Input: part model. Units: mm. Frame: model coordinates. A direction names the side the tool comes from. Coordinates: 2 decimals unless noted, no trailing zeros. Write each loop counter-clockwise with the first axis right and the second up, starting at its lowest first coordinate (ties: lowest second). Pieces come first, ordered by that corner, then holes. Notation, with made-up numbers: (-12.5, 3) - (10.5, 3) arc R37 ccw to (10.5, 41) - close; hole circle Ø1 at (16.25, 47.25). An arc over 180 degrees is marked (long way). Put each result on its own line as item: value. Start each with the question number.
1. Line query: line 1 (X direction, y = -1, z = -26.05); line 2 (Y direction, x = -23.25, z = -18); line 3 (Z direction, x = 24.5, y = -2.5). Output: solid intervals per line, ascending.
2. Cut plane B-B, the plane x = 24.1. Return loops of the section in (y, z), and give its area (3 significant figures).
3. Pin query (flat end, axial travel): pin 1 (4.5 mm diameter, centred on y = 0, z = -18, fed in from +X); pin 2 (3 mm diameter, centred on x = 24.1, z = 26.05, fed in from -Y). Return the tip coordinate at first contact, or that it passes through.
4. Access query for faces 1 (the cylindrical face through (-23.303, 0.125, 20.847)), 2 (the flat face through (19.5, 0, -18)), 3 (the cylindrical face through (19.601, -0.317, -24.142)). Directions: +Z, -Z, +X, -X, +Y, -Y. A direction counts if a zero-diameter tool reaches every point of the face in a straight line with its end or side. Return the directions, or none.
5. Cut plane C-C, the plane z = 18. Return loops of the section in (x, y), and give its area (3 significant figures).
6. Cut plane A-A, the plane z = -26.05. Return loops of the section in (x, y).
7. Pull-direction query (Z, two-part tool) for faces 4 (the flat face through (0, 0, 35)), 5 (the flat face through (0, 0, -35)), 6 (the cylindrical face through (-23.303, -0.125, -20.847)); classes: released by +Z, released by -Z, zero draft, split by the parting line, or undercut.
8. Cut plane D-D, the plane y = -2. Count the separate pieces of the cut face and the enclosed holes in it, and give its area (3 significant figures).
from build123d import *

# Parameters (mm, degrees)
SKETCH1_W           = 55
SKETCH1_H           = 70
SKETCH1_R           = 2
BOSS_EXTRUDE1_DEPTH = 5
SKETCH2_R           = 2.85
CUT_EXTRUDE1_DEPTH  = 8
CHAMFER1_SIZE       = 0.5


with BuildPart() as part:
    # Sketch1 → Boss-Extrude1 (new, symmetric)
    with BuildSketch(Plane(origin=(0, 0, 0), x_dir=(1, 0, 0), z_dir=(0, 1, 0))):
        Rectangle(SKETCH1_W, SKETCH1_H)
        with Locations(Location((24.1, -26.05, 0), (0, 0, 270))):
            Circle(SKETCH1_R, mode=Mode.SUBTRACT)
        with Locations(Location((-24.1, -24.75, 0), (0, 0, 270))):
            Circle(SKETCH1_R, mode=Mode.SUBTRACT)
        with Locations(Location((19, 26.05, 0), (0, 0, 270))):
            Circle(SKETCH1_R, mode=Mode.SUBTRACT)
        with Locations(Location((-8.9, 26.05, 0), (0, 0, 270))):
            Circle(SKETCH1_R, mode=Mode.SUBTRACT)
    extrude(amount=BOSS_EXTRUDE1_DEPTH, both=True)

    # Sketch2 → Cut-Extrude1 (cut)
    with BuildSketch(Plane(origin=(27.5, 0, 0), x_dir=(0, 0, -1), z_dir=(1, 0, 0))):
        with Locations((-18, 0)):
            Circle(SKETCH2_R)
        with Locations(Location((18, 0, 0), (0, 0, 180))):
            Circle(SKETCH2_R)
    cut_extrude1 = extrude(amount=-CUT_EXTRUDE1_DEPTH, mode=Mode.SUBTRACT)

    # Mirror1: Cut-Extrude1 across plane
    add(cut_extrude1.mirror(Plane(origin=(0, 0, 0), x_dir=(0, 0, 1), z_dir=(1, 0, 0))), mode=Mode.SUBTRACT)

    # Chamfer1
    chamfer1_edges = [part.edges().sort_by_distance(p)[0] for p in [
        (-24.1, 5, 22.75),
        (19, 5, -28.05),
        (24.1, 5, 24.05),
        (-8.9, 5, -28.05),
        (27.5, 0, 20.85),
        (27.5, 0, -20.85),
        (-27.5, 0, 20.85),
        (-27.5, 0, -20.85),
    ]]
    chamfer(chamfer1_edges, length=CHAMFER1_SIZE)


solid = part.part
Report:
1. line 1: x = -27.5 to -10.9, -6.9 to 17, 21 to 27.5
1. line 2: y = -5 to -2.85, 2.85 to 5
1. line 3: z = -35 to -19.37, -16.63 to 16.63, 19.37 to 24.09, 28.01 to 35
2. outline: (-5, -35) - (5, -35) - (5, 23.55) - (4.5, 24.05) - (-5, 24.05) - close; (-5, 28.05) - (4.5, 28.05) - (5, 28.55) - (5, 35) - (-5, 35) - close; hole circle Ø5.7 at (0, -18); hole circle Ø5.7 at (0, 18)
2. area: 609 mm^2
3. pin 1: stops at x = 19.5
3. pin 2: passes through
4. face 1: -X
4. face 2: +X
4. face 3: +Y, -Y
5. outline: (-27.5, -5) - (27.5, -5) - (27.5, -3.35) - (27, -2.85) - (19.5, -2.85) - (19.5, 2.85) - (27, 2.85) - (27.5, 3.35) - (27.5, 5) - (-27.5, 5) - (-27.5, 3.35) - (-27, 2.85) - (-19.5, 2.85) - (-19.5, -2.85) - (-27, -2.85) - (-27.5, -3.35) - close
5. area: 458 mm^2
6. outline: (-27.5, -5) - (-10.9, -5) - (-10.9, 4.5) - (-11.4, 5) - (-27.5, 5) - close; (-6.9, -5) - (17, -5) - (17, 4.5) - (16.5, 5) - (-6.4, 5) - (-6.9, 4.5) - close; (21, -5) - (27.5, -5) - (27.5, 5) - (21.5, 5) - (21, 4.5) - close
7. face 4: released by +Z
7. face 5: released by -Z
7. face 6: undercut
8. separate pieces: 1
8. enclosed holes: 4
8. area: 3,670 mm^2
